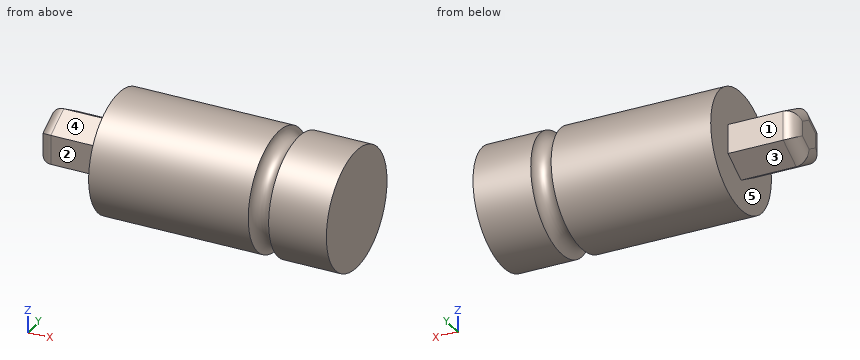
```python
from build123d import *

# Parameters (mm, degrees)
F0_R     = 11.1125
F1_DEPTH = 44.45
F3_DEPTH = 12.7
F4_R     = 2.38125
F6_R     = 1.905


with BuildPart() as f1:
    # F0 (on Right) → F1 (new body)
    with BuildSketch(Plane.YZ):
        Circle(F0_R)
    extrude(amount=F1_DEPTH)

    # F2 (on Right) → F3 (join)
    with BuildSketch(Plane.YZ):
        Polygon((-4.7625, 2.749631), (-4.7625, -2.749631), (0, -5.499261), (4.7625, -2.749631), (4.7625, 2.749631), (0, 5.499261), align=None)
    extrude(amount=-F3_DEPTH)

    # F4
    f4_edges = [f1.edges().sort_by_distance(p)[0] for p in [
        (-12.7, -2.38125, 4.124446),
        (-12.7, 2.38125, 4.124446),
        (-12.7, 4.7625, 0),
        (-12.7, 2.38125, -4.124446),
        (-12.7, -2.38125, -4.124446),
        (-12.7, -4.7625, 0),
    ]]
    fillet(f4_edges, radius=F4_R)

    # F6 (on Front) → F7 (revolve, cut)
    with BuildSketch(Plane.XZ):
        with Locations((31.75, 11.1125)):
            Circle(F6_R)
    revolve(axis=Axis((39.763745, 0, 0), (1, 0, 0)), mode=Mode.SUBTRACT)


solid = f1.part
```
Work out the finished part from the listing and answer in its coordinate system (mm). Face numbers are marked on the shaded views. A direction names the side the tool comes from. Give positions to 0.01 mm unless a question says otherwise; leave off trailing zeros. Order: outer loops, then holes, each group sorted by start corner. A loop starts at its lowest first (then second) coordinate and runs counter-clockwise, first axis right, second up. Notation, with made-up numbers: (-35.5, 10) - (5.5, 10) arc R38 cw to (5.5, 49) - close; hole circle Ø11 at (77.5, 60). An arc over 180 degrees is marked (long way). One line per item, written item: value. Start each with the question number.
1. Which of the six approach directions +Z, -Z, +X, -X, +Y, -Y give full straight-line access (tool end or side, diameter ignored) to the marked faces 1, 2, 3, 4 and 5?
2. Each of these flat-tipped pins is pushed along its axis until it touches: pin 1 Ø4 at (x, y) = (34.5, 8) entering from +Z; pin 2 Ø4.5 at (x, z) = (-6, -1.5) entering from +Y; pin 3 Ø4 at (x, z) = (36, 2.5) entering from -Y. Where does it stop, or does it pass through?
3. Consider line 1 (X direction, y = 8.5, z = -2); line 2 (X direction, y = 9.5, z = 0.5); line 3 (X direction, y = 5.25, z = -9.5). Determine where each line is inside the solid, lowest interval first.
4. Section B-B, the plane x = 26 is taken. Write down the section's boundary in (y, z) (1 decimal), then the cut area to 3 significant figures.
5. Section D-D, the plane x = 32.5 is taken. Write down the section's boundary in (y, z).
6. Section C-C, the plane x = -4 is taken. Write down the section's boundary in (y, z).
Filled sheet:
1. face 1: +Z, -Z, -X, +Y
1. face 2: +Z, -Z, -X, -Y
1. face 3: -Z, -X, +Y
1. face 4: +Z, -X, -Y
1. face 5: -X
2. pin 1: z = 9.35
2. pin 2: y = 4.76
2. pin 3: y = -11.1
3. line 1: 0 to 44.45
3. line 2: 0 to 30.72, 32.78 to 44.45
3. line 3: 0 to 29.86, 33.64 to 44.45
4. outline: circle Ø22.2 at (0, 0)
4. area: 388 mm²
5. outline: circle Ø18.72 at (0, 0)
6. outline: (-4.76, -2.75) - (0, -5.5) - (4.76, -2.75) - (4.76, 2.75) - (0, 5.5) - (-4.76, 2.75) - close
